Verification items for this drawing (mm, ordinates from the low corner). A direction names the side the tool comes from. Round coordinates to 2 decimals unless told otherwise and drop trailing zeros. Loops run counter-clockwise (first coordinate to the right, second up) from the corner with the lowest first, then second, coordinate; pieces in that order, holes last. Notation, with made-up numbers: (-3.75, 52.5) - (16.25, 52.5) arc R21 cw to (16.25, 90.5) - close; hole circle Ø8 at (86, -10.75). An arc over 180 degrees is marked (long way). Write item = value, one per line.
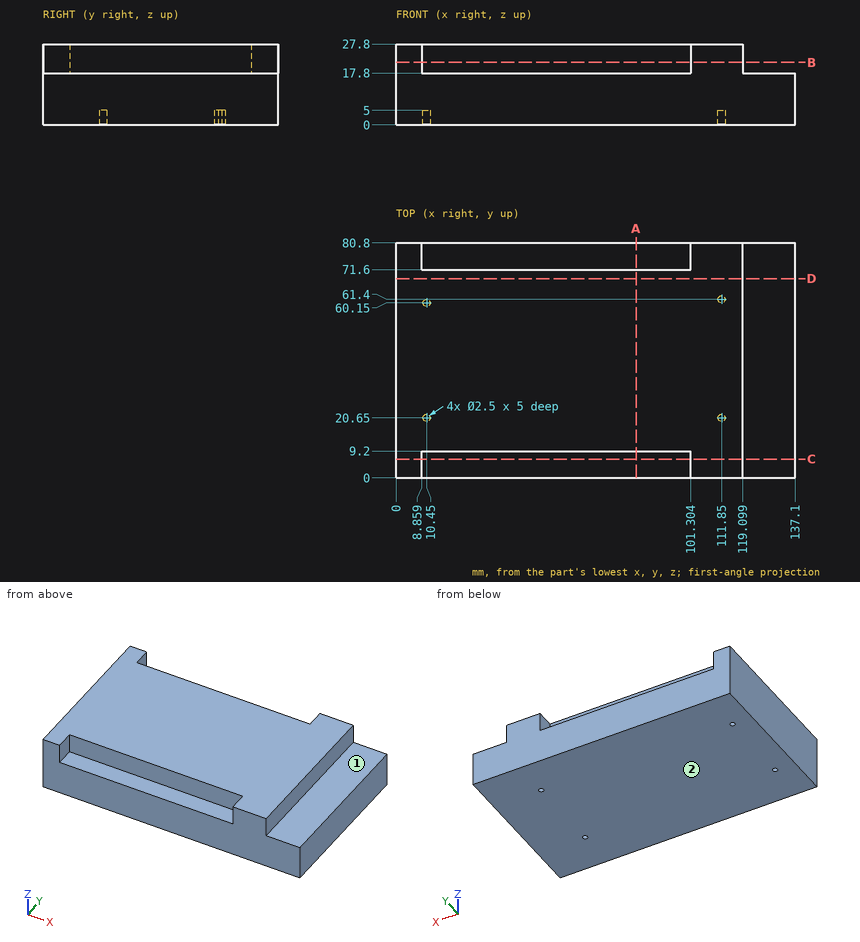
(1) Scan lines: L1, parallel to Y at x = 111.85, z = 3.8; L2, parallel to Y at x = 10.45, z = 2.95; L3, parallel to X at y = 9, z = 21.75. Record each from-to range of solid material in increasing order. Write a range as [from, to].
Answers follow:
L1 = [0, 19.4], [21.9, 60.15], [62.65, 80.8]
L2 = [0, 19.4], [21.9, 58.9], [61.4, 80.8]
L3 = [0, 8.86], [101.3, 119.1]
(2) Set-up check for the marked faces 1 and 2: record each of +Z, -Z, +X, -X, +Y, -Y from which the full face is reachable in a straight line by a thin tool's end or side.
Answers follow:
face_1 = +Z, +X, +Y, -Y
face_2 = -Z, +X, -X, +Y, -Y
(3) Section check D-D (y = 68.5). Enter the section's corners in (x, z).
Answers follow:
outline = (0, 0) - (137.1, 0) - (137.1, 17.8) - (119.1, 17.8) - (119.1, 27.8) - (0, 27.8) - close
(4) Section check B-B (z = 21.5). Enter the section's corners in (x, y), then the cut area to 3 significant figures.
Answers follow:
outline = (0, 0) - (8.86, 0) - (8.86, 9.2) - (101.3, 9.2) - (101.3, 0) - (119.1, 0) - (119.1, 80.8) - (101.3, 80.8) - (101.3, 71.6) - (8.86, 71.6) - (8.86, 80.8) - (0, 80.8) - close
area = 7,920 mm²
(5) Gauge pin test, flat ends, axial feed: pin 1 (3 mm diameter, centred on x = 40, z = 20.5, fed in from +Y); pin 2 (4.5 mm diameter, centred on x = 72, y = 2.5, fed in from +Z); pin 3 (1.2 mm diameter, centred on x = 112, y = 20.5, fed in from -Z). Record the tip position at first contact, or that the pin passes through.
Answers follow:
pin_1 = 71.6
pin_2 = 17.8
pin_3 = 5
(6) Section check A-A (x = 82.5). Enter the section's corners in (y, z).
Answers follow:
outline = (0, 0) - (80.8, 0) - (80.8, 17.8) - (71.6, 17.8) - (71.6, 27.8) - (9.2, 27.8) - (9.2, 17.8) - (0, 17.8) - close
(7) Section check C-C (y = 6.5). Enter the section's corners in (x, z).
Answers follow:
outline = (0, 0) - (137.1, 0) - (137.1, 17.8) - (119.1, 17.8) - (119.1, 27.8) - (101.3, 27.8) - (101.3, 17.8) - (8.86, 17.8) - (8.86, 27.8) - (0, 27.8) - close
